Geometry check sheet. Reference: the model listing, model coordinates, mm. A direction names the side the tool comes from. Coordinates: 2 decimals unless noted, no trailing zeros. Loops run counter-clockwise (first coordinate to the right, second up) from the corner with the lowest first, then second, coordinate; pieces in that order, holes last.
from build123d import *

# Parameters (mm, degrees)
SKETCH1_W            = 60
SKETCH1_H            = 50
BOSS_EXTRUDE1_DEPTH  = 200
SKETCH2_W            = 120
SKETCH2_H            = 50
BOSS_EXTRUDE2_DEPTH  = 2.5
FILLET1_R            = 10
SKETCH3_R            = 5
CUT_EXTRUDE1_DEPTH   = 403.779406127
FILLET1_OF_MIRROR1_R = 10
SKETCH4_W            = 50
SKETCH4_H            = 40
CUT_EXTRUDE2_DEPTH   = 411.18288604


with BuildPart() as part:
    # Sketch1 → Boss-Extrude1 (new, symmetric)
    with BuildSketch(Plane(origin=(0, 0, 0), x_dir=(-1, 0, 0), z_dir=(0, 1, 0))):
        Rectangle(SKETCH1_W, SKETCH1_H)
    extrude(amount=BOSS_EXTRUDE1_DEPTH, both=True)

    # Sketch2 → Boss-Extrude2 (add, symmetric)
    with BuildSketch(Plane(origin=(0, 200, 0), x_dir=(-1, 0, 0), z_dir=(0, 1, 0))):
        Rectangle(SKETCH2_W, SKETCH2_H)
    boss_extrude2 = extrude(amount=BOSS_EXTRUDE2_DEPTH, both=True)

    # Fillet1
    fillet1_edges = [part.edges().sort_by_distance(p)[0] for p in [
        (-30, 197.5, 0),
        (30, 197.5, 0),
    ]]
    fillet(fillet1_edges, radius=FILLET1_R)

    # Sketch3 → Cut-Extrude1 (cut, through all)
    with BuildSketch(Plane.XZ.offset(-197.5)):
        with Locations(Location((50, 15, 0), (0, 0, 270))):
            Circle(SKETCH3_R)
        with Locations(Location((50, -15, 0), (0, 0, 90))):
            Circle(SKETCH3_R)
        with Locations(Location((-50, 15, 0), (0, 0, 90))):
            Circle(SKETCH3_R)
        with Locations(Location((-50, -15, 0), (0, 0, 270))):
            Circle(SKETCH3_R)
    cut_extrude1 = extrude(amount=-CUT_EXTRUDE1_DEPTH, mode=Mode.SUBTRACT)

    # Mirror1: Boss-Extrude2, Cut-Extrude1 across plane
    add(boss_extrude2.mirror(Plane.ZX))
    add(cut_extrude1.mirror(Plane.ZX), mode=Mode.SUBTRACT)

    # Fillet1 of Mirror1
    fillet1_of_mirror1_edges = [part.edges().sort_by_distance(p)[0] for p in [
        (-30, -197.5, 0),
        (30, -197.5, 0),
    ]]
    fillet(fillet1_of_mirror1_edges, radius=FILLET1_OF_MIRROR1_R)

    # Sketch4 → Cut-Extrude2 (cut, through all)
    with BuildSketch(Plane.XZ.offset(202.5)):
        Rectangle(SKETCH4_W, SKETCH4_H)
    extrude(amount=-CUT_EXTRUDE2_DEPTH, mode=Mode.SUBTRACT)


solid = part.part
(1) Sectioned sample at B-B on y = -16. Record the cut outline in (x, z).
Findings:
outline: (-30, -25) - (30, -25) - (30, 25) - (-30, 25) - close; hole (-25, -20) - (25, -20) - (25, 20) - (-25, 20) - close
(2) Gauge pin test, flat ends, axial feed: pin 1 Ø5 at (y, z) = (-153.5, 15.5) entering from +X; pin 2 Ø6 at (x, z) = (-50, 15) entering from +Y; pin 3 Ø8 at (y, z) = (-53, 11) entering from -X. Record the tip position at first contact, or that the pin passes through.
Findings:
pin 1: stops at x = 30
pin 2: passes through
pin 3: stops at x = -30
(3) Draft check along Y on faces 1 (the flat face through (1, -202.5, -22)), 2 (the flat face through (-25, -3, 0)), 3 (the flat face through (-50, -197.5, 0)), 4 (the flat face through (-30, 3, 0)). Enter one of: +Y half, -Y half, draft (parallel to the pull), parting line (faces both ways), or undercut.
Findings:
face 1: -Y half
face 2: draft
face 3: undercut
face 4: undercut
(4) Sectioned sample at C-C on x = 50. Record the cut outline in (y, z).
Findings:
outline: (-202.5, -25) - (-197.5, -25) - (-197.5, -20) - (-202.5, -20) - close; (-202.5, -10) - (-197.5, -10) - (-197.5, 10) - (-202.5, 10) - close; (-202.5, 20) - (-197.5, 20) - (-197.5, 25) - (-202.5, 25) - close; (197.5, -25) - (202.5, -25) - (202.5, -20) - (197.5, -20) - close; (197.5, -10) - (202.5, -10) - (202.5, 10) - (197.5, 10) - close; (197.5, 20) - (202.5, 20) - (202.5, 25) - (197.5, 25) - close
(5) Access from +Z, -Z, +X, -X, +Y, -Y to the whole of each face (thin tool, end or side, straight path). Record for faces 5 (the cylindrical face through (33.01, -194.65, -0.35)), 6 (the cylindrical face through (-32.85, -194.49, -0.35)), 7 (the flat face through (0, -3, 20)).
Findings:
face 5: +Z, -Z, +X
face 6: +Z, -Z, -X
face 7: +Y, -Y
(6) Sectioned sample at A-A on x = -1.5. Record the cut outline in (y, z).
Findings:
outline: (-202.5, -25) - (202.5, -25) - (202.5, -20) - (-202.5, -20) - close; (-202.5, 20) - (202.5, 20) - (202.5, 25) - (-202.5, 25) - close
(7) Sectioned sample at D-D on z = 15. State how many separate pieces and enclosed holes the cut face has, and give its area (3 significant figures).
Findings:
separate pieces: 6
enclosed holes: 0
area: 4,540 mm2
(8) Scan lines: L1, parallel to X at y = 199.45, z = -15; L2, parallel to Z at x = -16.5, y = 6.5; L3, parallel to Z at x = -50, y = -201. Record each from-to range of solid material in increasing order.
Findings:
L1: x = -60 to -55, -45 to -25, 25 to 45, 55 to 60
L2: z = -25 to -20, 20 to 25
L3: z = -25 to -20, -10 to 10, 20 to 25
